Model file for the job. Use its own axes, mm. Face numbers are marked on the shaded views. A direction names the side the tool comes from. Round coordinates to 2 decimals unless told otherwise and drop trailing zeros. Order: outer loops, then holes, each group sorted by start corner. A loop starts at its lowest first (then second) coordinate and runs counter-clockwise, first axis right, second up. Notation, with made-up numbers: (14, 80) -> (37, 80) arc R18 cw to (37, 87) -> close; hole circle Ø7 at (81.25, -38.5). An arc over 180 degrees is marked (long way). Put each result on its own line as item: value. Start each with the question number.
Q1. Flat gauge pins, fed straight in: P1, Ø1.8, axis at x = -2.5, y = 16, coming from the -Z side; P2, Ø4, axis at x = -22.86, y = 2.54, coming from the -Z side; P3, Ø12, axis at x = -31, z = 5.5, coming from the -Y side; P4, Ø1.2, axis at y = 8, z = 4, coming from the -X side. Where does each tip first touch, or does it go through?
Q2. Probe L1, parallel to Y at x = -2, z = 2; L2, parallel to Z at x = -2.54, y = 45.2; L3, parallel to Y at x = -22.86, z = 1.7. List the from-to ranges inside material, lowest first.
Q3. 3-axis set-ups, long thin cutter, end or side, ignore diameter. For the marked faces 1, 2 and 3: which of +Z, -Z, +X, -X, +Y, -Y reach the whole face in a straight line?
Q4. Cut at A-A, the plane y = 44.5. List the corners of the cut face in (x, z), and give its area (3 significant figures).
Q5. Cut at B-B, the plane x = -11.5. List the corners of the cut face in (y, z), and give its area (3 significant figures).
from build123d import *

# Parameters (mm, degrees)
SKIZZE1_R                         = 3
AUFSATZ_LINEAR_AUSTRAGEN1_DEPTH   = 5
AUFSATZ_LINEAR_AUSTRAGEN1_2_DEPTH = 5
AUFSATZ_LINEAR_AUSTRAGEN1_3_DEPTH = 5
SKIZZE3_R                         = 3
SKIZZE6_W                         = 20.32
SKIZZE6_H                         = 6
AUFSATZ_LINEAR_AUSTRAGEN2_DEPTH   = 4
AUFSATZ_LINEAR_START              = -5
SKIZZE8_W                         = 6
SKIZZE8_H                         = 12.7
AUFSATZ_LINEAR_AUSTRAGEN3_DEPTH   = 4
AUFSATZ_LINEAR_AUSTRAGEN4_DEPTH   = 4
SKIZZE14_R                        = 3
SCHNITT_LINEAR_AUSTRAGEN2_DEPTH   = 48.39873951
SKIZZE16_R                        = 1.7
SCHNITT_LINEAR_AUSTRAGEN3_DEPTH   = 4
SKIZZE17_R                        = 1.7
SCHNITT_LINEAR_AUSTRAGEN4_DEPTH   = 4
SCHNITT_LINEAR_AUSTRAGEN6_DEPTH   = 4


with BuildPart() as part:
    # Skizze1 → Aufsatz-Linear austragen1 (new body)
    with BuildSketch(Plane.XY):
        with Locations((-2.54, 15.24)):
            Circle(SKIZZE1_R)
    extrude(amount=AUFSATZ_LINEAR_AUSTRAGEN1_DEPTH)



with BuildPart() as body_2:
    # Skizze1 → Aufsatz-Linear austragen1 2 (new body)
    with BuildSketch(Plane.XY):
        with Locations((-2.54, 2.54)):
            Circle(SKIZZE1_R)
    extrude(amount=AUFSATZ_LINEAR_AUSTRAGEN1_2_DEPTH)



with BuildPart() as body_3:
    # Skizze1 → Aufsatz-Linear austragen1 3 (new body)
    with BuildSketch(Plane.XY):
        with Locations((-22.86, 2.54)):
            Circle(SKIZZE1_R)
    extrude(amount=AUFSATZ_LINEAR_AUSTRAGEN1_3_DEPTH)


with BuildPart() as body_4:
    # Austragung1: sweep along a path in Skizze2
    with BuildLine(Plane(origin=(0, 0, 0), x_dir=(0, 0, -1), z_dir=(1, 0, 0))) as austragung1_path:
        Line((-21.93, 46.93873951), (-21.93, 33.848580958))
        ThreePointArc((-21.93, 33.848580958), (-21.752467402, 31.972645421), (-21.226173172, 30.163317826))
        Line((-21.226173172, 30.163317826), (-15.296173172, 15.204736868))
        ThreePointArc((-15.296173172, 15.204736868), (-11.619046569, 10.617979953), (-6, 8.89))
        Line((-6, 8.89), (-5, 8.89))
    # Skizze3 → Austragung1 (sweep)
    with BuildSketch(Plane.XY.offset(5)):
        with Locations((-2.54, 8.89)):
            Circle(SKIZZE3_R)
    sweep(path=austragung1_path.line)


with BuildPart() as body_2_1:
    add(body_2.part)

    add(body_3.part)  # Aufsatz-Linear austragen2 merges body 3
    # Skizze6 → Aufsatz-Linear austragen2 (add)
    with BuildSketch(Plane.XY.offset(5)):
        with Locations((-12.7, 2.54)):
            Rectangle(SKIZZE6_W, SKIZZE6_H)
    extrude(amount=-AUFSATZ_LINEAR_AUSTRAGEN2_DEPTH)


with BuildPart() as part_1:
    add(part.part)

    add(body_2_1.part)  # Aufsatz-Linear austragen3 merges body 2

    add(body_4.part)  # Aufsatz-Linear austragen3 merges body 4
    # Skizze8 → Aufsatz-Linear austragen3 (add)
    with BuildSketch(Plane(origin=(0, 0, 0), x_dir=(-1, 0, 0), z_dir=(0, 0, -1)).offset(AUFSATZ_LINEAR_START)):
        with Locations((2.54, 8.89)):
            Rectangle(SKIZZE8_W, SKIZZE8_H)
    extrude(amount=AUFSATZ_LINEAR_AUSTRAGEN3_DEPTH)

    # Skizze9 → Aufsatz-Linear austragen4 (add)
    with BuildSketch(Plane(origin=(0, 0, 0), x_dir=(-1, 0, 0), z_dir=(0, 0, -1)).offset(AUFSATZ_LINEAR_START)):
        Polygon((4.12999682, 17.783994912), (0.95000318, 12.696005088), (21.27000318, -0.003994912), (24.44999682, 5.083994912), align=None)
    extrude(amount=AUFSATZ_LINEAR_AUSTRAGEN4_DEPTH)

    # Austragung3: sweep along a path in Skizze12
    with BuildLine(Plane(origin=(-70.149644345, 31.847131815, -6.332474017), x_dir=(0.978512631, 0, 0.206186883), z_dir=(0.206186883, 0, -0.978512631))) as austragung3_path:
        Line((-6.001962715, -15.091607694), (-6.001962715, -10.091607694))
        ThreePointArc((-6.001962715, -10.091607694), (5.537660917, 17.767508183), (33.396776795, 29.307131815))
        Line((33.396776795, 29.307131815), (44.6436495, 29.307131815))
        Line((44.6436495, 29.307131815), (59.6436495, 29.307131815))
    # Skizze14 → Austragung3 (sweep)
    with BuildSketch(Plane(origin=(0, 46.93873951, 0), x_dir=(-1, 0, 0), z_dir=(0, -1, 0))):
        with Locations((76.022640673, 7.57)):
            Circle(SKIZZE14_R)
    sweep(path=austragung3_path.line)

    # Skizze15 → Schnitt-Linear austragen2 (cut, through all)
    with BuildSketch(Plane(origin=(0, -0.46, 0), x_dir=(-1, 0, 0), z_dir=(0, -1, 0))):
        Polygon((11.584184705, -5), (12.406140588, -8.900802043), (30.918395198, -5), align=None)
    extrude(amount=-SCHNITT_LINEAR_AUSTRAGEN2_DEPTH, mode=Mode.SUBTRACT)

    # Skizze16 → Schnitt-Linear austragen3 (cut)
    with BuildSketch(Plane(origin=(0, 46.93873951, 0), x_dir=(1, 0, 0), z_dir=(0, 1, 0))):
        with Locations((-2.54, -21.93)):
            Circle(SKIZZE16_R)
        with Locations((-76.022640673, 7.57)):
            Circle(SKIZZE16_R)
    extrude(amount=-SCHNITT_LINEAR_AUSTRAGEN3_DEPTH, mode=Mode.SUBTRACT)

    # Skizze17 → Schnitt-Linear austragen4 (cut)
    with BuildSketch(Plane(origin=(0, 0, 0), x_dir=(-1, 0, 0), z_dir=(0, 0, -1))):
        with Locations((2.54, 2.54)):
            Circle(SKIZZE17_R)
        with Locations((2.54, 15.24)):
            Circle(SKIZZE17_R)
        with Locations((22.86, 2.54)):
            Circle(SKIZZE17_R)
    extrude(amount=-SCHNITT_LINEAR_AUSTRAGEN4_DEPTH, mode=Mode.SUBTRACT)

    # Skizze19 → Schnitt-Linear austragen6 (cut)
    with BuildSketch(Plane(origin=(0, 0, 1), x_dir=(-1, 0, 0), z_dir=(0, 0, -1))):
        with BuildLine():
            Line((4.872034586, 17.320221308), (23.707959054, 5.547768516))
            ThreePointArc((23.707959054, 5.547768516), (12.505452744, 8.57872439), (4.872034586, 17.320221308))
        make_face()
    extrude(amount=-SCHNITT_LINEAR_AUSTRAGEN6_DEPTH, mode=Mode.SUBTRACT)


solid = part_1.part
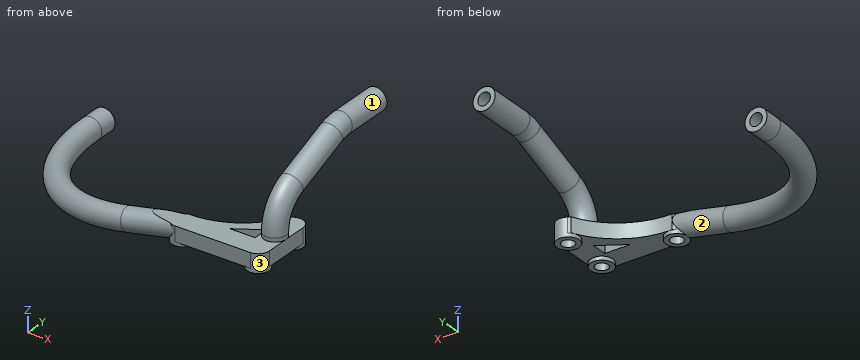
Ans:
1. P1: stops at z = 4
1. P2: stops at z = 0
1. P3: stops at y = -0.46
1. P4: stops at x = -14.68
2. L1: y = -0.41 to 0.93, 4.15 to 13.63, 16.85 to 18.19
2. L2: z = 18.93 to 20.23, 23.63 to 24.93
2. L3: y = -0.46 to 0.84, 4.24 to 5.54
3. face 1: +Y
3. face 2: none
3. face 3: -Z
4. outline: circle Ø6 at (-76.02, -7.57); circle Ø6 at (-2.54, 21.93); hole circle Ø3.4 at (-76.02, -7.57); hole circle Ø3.4 at (-2.54, 21.93)
4. area: 38.4 mm^2
5. outline: (-0.46, 1) -> (5.54, 1) -> (5.54, 5) -> (-0.46, 5) -> close; (6.1, 1) -> (9.25, 1) -> (9.25, 5) -> (6.1, 5) -> close
5. area: 36.6 mm^2
